Could you check a few things on this model? Use its own coordinates, in mm. A direction names the side the tool comes from. Give positions to 0.01 mm unless a question says otherwise; leave off trailing zeros. Loops run counter-clockwise (first coordinate to the right, second up) from the corner with the lowest first, then second, coordinate; pieces in that order, holes last. Notation, with made-up numbers: M 20,59 L 53,59 A22 cw 53,78 Z; hole C 58.5,24.25 d10. An arc over 180 degrees is marked long. Write each question's results on one line, items separated by ' | '. Start each with the question number.
from build123d import *

# Parameters (mm, degrees)
SKETCH5_R              = 1.85
CUT_EXTRUDE2_DEPTH     = 6
CUT_EXTRUDE3_START     = -6
SKETCH8_R              = 1.85
CUT_EXTRUDE3_DEPTH     = 6
CHAMFER1_SIZE          = 0.3
CUT_EXTRUDE4_START     = 10.763479818
CUT_EXTRUDE4_OUTLINE_R = 2.5
CUT_EXTRUDE4_DEPTH     = 13.236520282


# Read off the part's stored shape, not the designer's step: Cut-Extrude4
with BuildPart() as part:
    # Sketch1 → Revolve1 (revolve)
    with BuildSketch(Plane.XY, mode=Mode.PRIVATE) as revolve1_sk:
        Polygon((-14.05, 0), (-24, 0), (-24, 31.5), (-14.05, 31.5), (-14.05, 29.3), (-16.3, 29.3), (-16.3, 25.2), (-14.05, 25.2), (-14.05, 23.5), (-14.55, 23.5), (-14.55, 23), (-14.05, 23), (-11.05, 23), (-11.05, 8.5), (-14.05, 8.5), (-14.55, 8.5), (-14.55, 8), (-14.05, 8), (-14.05, 6.3), (-16.3, 6.3), (-16.3, 2.2), (-14.05, 2.2), align=None)
    revolve(revolve1_sk.sketch.rotate(Axis((0, 0, 0), (0, 1, 0)), 270), axis=Axis((0, 0, 0), (0, 1, 0)))

    # Sketch5 → Cut-Extrude2 (cut)
    with BuildSketch(Plane(origin=(0, 31.5, 0), x_dir=(1, 0, 0), z_dir=(0, 1, 0))):
        with Locations(Location((-20, 0, 0), (0, 0, 270))):
            Circle(SKETCH5_R)
        with Locations(Location((-10, 17.320508076, 0), (0, 0, 270))):
            Circle(SKETCH5_R)
        with Locations(Location((10, 17.320508076, 0), (0, 0, 270))):
            Circle(SKETCH5_R)
        with Locations(Location((20, 0, 0), (0, 0, 270))):
            Circle(SKETCH5_R)
        with Locations(Location((10, -17.320508076, 0), (0, 0, 270))):
            Circle(SKETCH5_R)
        with Locations(Location((-10, -17.320508076, 0), (0, 0, 270))):
            Circle(SKETCH5_R)
    extrude(amount=-CUT_EXTRUDE2_DEPTH, mode=Mode.SUBTRACT)

    # Sketch8 → Cut-Extrude3 (cut)
    with BuildSketch(Plane.XZ.offset(CUT_EXTRUDE3_START)):
        with Locations(Location((-20, 0, 0), (0, 0, 90))):
            Circle(SKETCH8_R)
        with Locations(Location((-10, 17.320508076, 0), (0, 0, 90))):
            Circle(SKETCH8_R)
        with Locations(Location((10, 17.320508076, 0), (0, 0, 90))):
            Circle(SKETCH8_R)
        with Locations(Location((20, 0, 0), (0, 0, 90))):
            Circle(SKETCH8_R)
        with Locations(Location((10, -17.320508076, 0), (0, 0, 90))):
            Circle(SKETCH8_R)
        with Locations(Location((-10, -17.320508076, 0), (0, 0, 90))):
            Circle(SKETCH8_R)
    extrude(amount=CUT_EXTRUDE3_DEPTH, mode=Mode.SUBTRACT)

    # Chamfer1
    chamfer1_edges = [part.edges().sort_by_distance(p)[0] for p in [
        (0, 2.2, 14.05),
        (0, 0, 24),
        (0, 31.5, 24),
        (0, 31.5, 14.05),
        (0, 29.3, 14.05),
        (0, 25.2, 14.05),
        (-20, 31.5, -1.85),
        (-10, 31.5, 15.470508076),
        (10, 31.5, 15.470508076),
        (20, 31.5, -1.85),
        (10, 31.5, -19.170508076),
        (-10, 31.5, -19.170508076),
        (-20, 0, -1.85),
        (-10, 0, -19.170508076),
        (10, 0, -19.170508076),
        (20, 0, -1.85),
        (10, 0, 15.470508076),
        (-10, 0, 15.470508076),
    ]]
    chamfer(chamfer1_edges, length=CHAMFER1_SIZE)

    # Cut-Extrude4 outline → Cut-Extrude4 (cut)
    with BuildSketch(Plane.XY.offset(CUT_EXTRUDE4_START)):
        with Locations((0, 15.6)):
            Circle(CUT_EXTRUDE4_OUTLINE_R)
    extrude(amount=CUT_EXTRUDE4_DEPTH, mode=Mode.SUBTRACT)


solid = part.part
1) Which directions (+Z, -Z, +X, -X, +Y, -Y) give clear straight access to the entire face, cutting with the end or side of a thin tool? Please do faces 1 (the face through (-20, 6, 0)), 2 (the face through (9.918, 27.221, 12.935)), 3 (the face through (9.29, 28.39, 19.03)), 4 (the face through (4.23, 15.65, -10.21)).
2) Thinking about a two-plate mould opening in Y: for faces 5 (the face through (20, 6, 0)), 6 (the face through (11, 25.2, -10)), 7 (the face through (12.465, 7.138, -6.483)), which applies, pulls with the +Y half, pulls with the -Y half, needs draft (parallel to the pull), parting line crosses it, or undercut?
3) Please list where these lines run through material, in increasing order: line 1 (Y direction, x = 5.5, z = 15); line 2 (X direction, y = 12.5, z = 0); line 3 (X direction, y = 8.4, z = 0). Write a range as from..to.
4) If we section it at A-A on y = 4.5: Write out the boundary of the cut face in (x, z), plus the area to 3 significant figures.
5) If we section it at D-D on y = 15.6: Write out the boundary of the cut face in (x, z), plus the area to 3 significant figures.
6) I'm going to push flat-ended pins straight in: P1, Ø5, axis at y = 11, z = 10, coming from the +X side; P2, Ø1.1, axis at x = -19, z = 0, coming from the -Y side; P3, Ø2, axis at y = 22.5, z = 3, coming from the +X side; P4, Ø6, axis at x = -11.5, z = 11, coming from the -Y side. Where does each tip first touch, or does it pass through?
7) If we section it at B-B on x = 0: State how many separate pieces and enclosed holes the cut face has, plus the area to 3 significant figures.
8) If we section it at C-C on y = 20.5: Write out the boundary of the cut face in (x, z).
Calculated:
1) face 1: -Y | face 2: none | face 3: +Y | face 4: +Y, -Y
2) face 5: pulls with the -Y half | face 6: undercut | face 7: needs draft
3) line 1: y = 0..2.2, 6.3..25.2, 29.3..31.5 | line 2: x = -24..-11.05, 11.05..24 | line 3: x = -24..-14.55, 14.55..24
4) outline: C 0,0 d48; hole C -20,0 d3.7; hole C 0,0 d32.6; hole C -10,-17.32 d3.7; hole C -10,17.32 d3.7; hole C 10,-17.32 d3.7; hole C 10,17.32 d3.7; hole C 20,0 d3.7 | area: 910 mm2
5) outline: M -2.5,10.76 L -2.5,23.87 A24 ccw long 2.5,23.87 L 2.5,10.76 A11.05 cw long Z | area: 1,360 mm2
6) P1: stops at x = 22.8 | P2: stops at y = 6 | P3: stops at x = 23.92 | P4: stops at y = 0
7) separate pieces: 3 | enclosed holes: 0 | area: 611 mm2
8) outline: C 0,0 d48; hole C 0,0 d22.1
